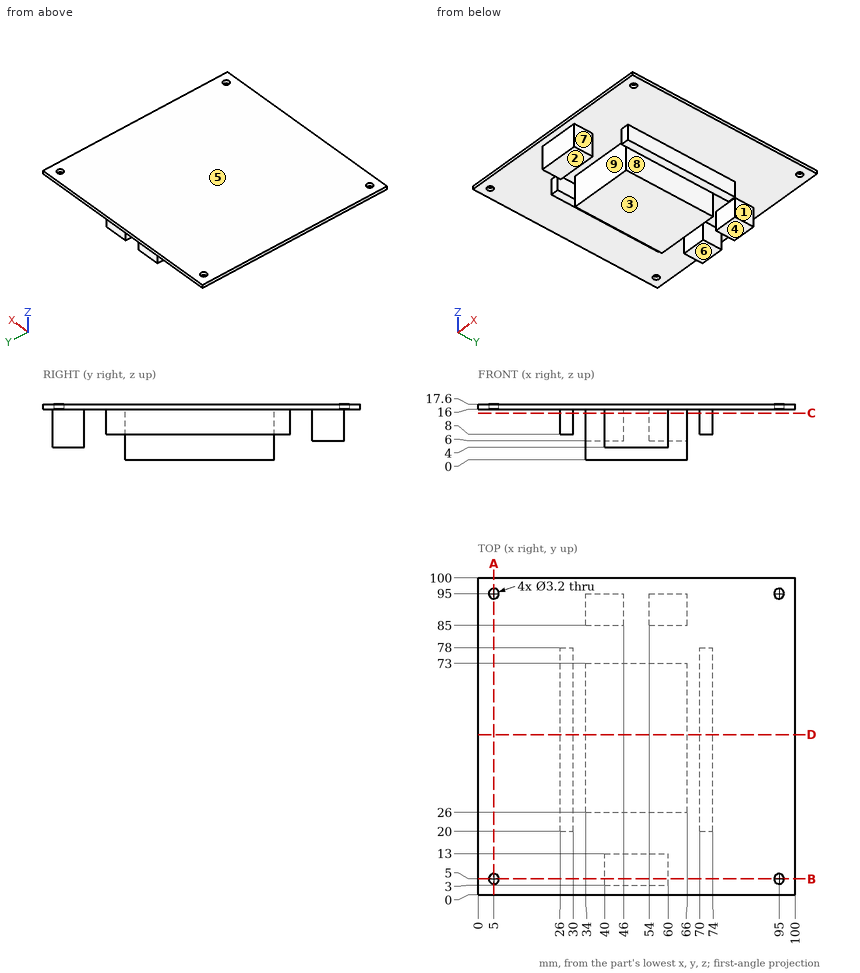
Geometry: see drawing. Coordinates: mm, zero at the bounding-box minimum. A direction names the side the tool comes from. Give positions to 0.01 mm unless a question says otherwise; leave off trailing zeros. Order: outer loops, then holes, each group sorted by start corner. A loop starts at its lowest first (then second) coordinate and runs counter-clockwise, first axis right, second up.
1. Pin query (flat end, axial travel): pin 1 Ø4.5 at (x, y) = (27, 63.5) entering from -Z; pin 2 Ø2.5 at (y, z) = (49.5, 13) entering from +X; pin 3 Ø5 at (x, z) = (61, 10.5) entering from +Y; pin 4 Ø1 at (y, z) = (79.5, 6.5) entering from +X. Return the tip coordinate at first contact, or that it passes through.
Computed:
pin 1: stops at z = 8
pin 2: stops at x = 74
pin 3: stops at y = 95
pin 4: passes through
2. Cut plane C-C (z = 14.75). Return loops of the section in (x, y).
Computed:
outline: (26, 20) - (30, 20) - (30, 78) - (26, 78) - close; (34, 26) - (66, 26) - (66, 73) - (34, 73) - close; (34, 85) - (46, 85) - (46, 95) - (34, 95) - close; (40, 3) - (60, 3) - (60, 13) - (40, 13) - close; (54, 85) - (66, 85) - (66, 95) - (54, 95) - close; (70, 20) - (74, 20) - (74, 78) - (70, 78) - close
3. Draft query along X for the marked faces 6, 7, 8 and 9. Return one class per face: released by +X, released by -X, zero draft, split by the parting line, or undercut.
Computed:
face 6: zero draft
face 7: released by +X
face 8: undercut
face 9: undercut
4. Cut plane A-A (x = 5). Return loops of the section in (y, z), and give its area (3 significant figures).
Computed:
outline: (0, 16) - (3.4, 16) - (3.4, 17.6) - (0, 17.6) - close; (6.6, 16) - (93.4, 16) - (93.4, 17.6) - (6.6, 17.6) - close; (96.6, 16) - (100, 16) - (100, 17.6) - (96.6, 17.6) - close
area: 150 mm2
5. Cut plane B-B (y = 5). Return loops of the section in (x, z).
Computed:
outline: (0, 16) - (3.4, 16) - (3.4, 17.6) - (0, 17.6) - close; (6.6, 16) - (40, 16) - (40, 4) - (60, 4) - (60, 16) - (93.4, 16) - (93.4, 17.6) - (6.6, 17.6) - close; (96.6, 16) - (100, 16) - (100, 17.6) - (96.6, 17.6) - close
6. Line query: probe 1 along Y at (x, z) = (5, 17.15); probe 2 along Y at (x, z) = (45.5, 14.75); probe 3 along X at (y, z) = (30, 15.25). Output: solid intervals per line, ascending.
Computed:
probe 1: y = 0 to 3.4, 6.6 to 93.4, 96.6 to 100
probe 2: y = 3 to 13, 26 to 73, 85 to 95
probe 3: x = 26 to 30, 34 to 66, 70 to 74
7. Cut plane D-D (y = 50.5). Return loops of the section in (x, z), and give its area (3 significant figures).
Computed:
outline: (0, 16) - (26, 16) - (26, 8) - (30, 8) - (30, 16) - (34, 16) - (34, 0) - (66, 0) - (66, 16) - (70, 16) - (70, 8) - (74, 8) - (74, 16) - (100, 16) - (100, 17.6) - (0, 17.6) - close
area: 736 mm2
8. Set-up query: the marked faces 1, 2, 3, 4 and 5. Return all of +Z, -Z, +X, -X, +Y, -Y with unobstructed straight access to the full face (end or side cutting, diameter ignored); none if empty.
Computed:
face 1: -Z, +X, +Y, -Y
face 2: -Z, +X, -X, -Y
face 3: -Z, +X, -X, +Y, -Y
face 4: -Z, +X, -X, +Y
face 5: +Z, +X, -X, +Y, -Y
